```python
from build123d import *

# Parameters (mm, degrees)
SKIZZE1_W                       = 50
SKIZZE1_H                       = 2
SKIZZE1_W_2                     = 2
SKIZZE1_H_2                     = 48
AUFSATZ_LINEAR_AUSTRAGEN1_DEPTH = 30
AUFSATZ_LINEAR_AUSTRAGEN2_DEPTH = 30
SKIZZE3_R                       = 1.5
SCHNITT_LINEAR_AUSTRAGEN1_DEPTH = 30


with BuildPart() as part:
    # Skizze1 → Aufsatz-Linear austragen1 (new body)
    with BuildSketch(Plane.XY):
        with Locations((-2.795178436, 3.083333333)):
            Rectangle(SKIZZE1_W, SKIZZE1_H)
        with Locations((21.204821564, -21.916666667)):
            Rectangle(SKIZZE1_W_2, SKIZZE1_H_2)
    extrude(amount=AUFSATZ_LINEAR_AUSTRAGEN1_DEPTH)

    # Skizze2 → Aufsatz-Linear austragen2 (add)
    with BuildSketch(Plane.XY.offset(30)):
        Polygon((15.215533088, 2.083333333), (20.204821564, -2.916666667), (20.204821564, 2.083333333), align=None)
    extrude(amount=-AUFSATZ_LINEAR_AUSTRAGEN2_DEPTH)

    # Skizze3 → Schnitt-Linear austragen1 (cut)
    with BuildSketch(Plane(origin=(8.665746428, 8.647181758, 0), x_dir=(0, 0, 1), z_dir=(-0.7078646055315657, -0.7063481437900443, 0))):
        with Locations(Location((15, -12.806243307, 0), (0, 0, 270))):
            Circle(SKIZZE3_R)
    extrude(amount=-SCHNITT_LINEAR_AUSTRAGEN1_DEPTH, mode=Mode.SUBTRACT)


solid = part.part
```
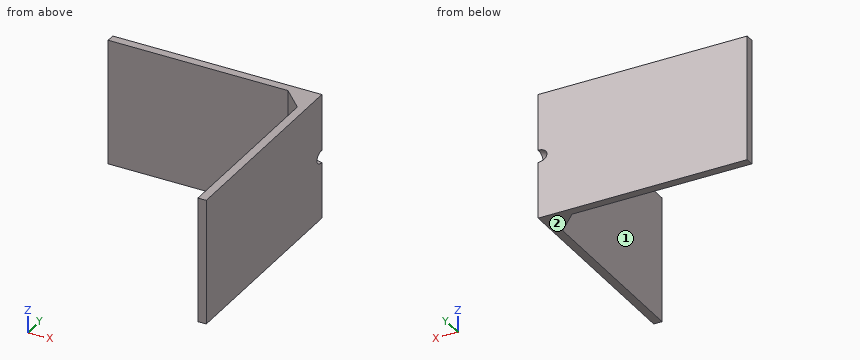
The model under review builds one solid part; all positions refer to its coordinate system, in mm. Face numbers are marked on the shaded views. A direction names the side the tool comes from. Round coordinates to 2 decimals unless told otherwise and drop trailing zeros. Write each loop counter-clockwise with the first axis right and the second up, starting at its lowest first coordinate (ties: lowest second). Pieces come first, ordered by that corner, then holes. Notation, with made-up numbers: (-15.75, 74.5) - (19.25, 74.5) arc R17 cw to (19.25, 87.5) - close; hole circle Ø9 at (52, 48.5). An arc over 180 degrees is marked (long way). One line per question, with ' | ' between items.
Item 1: For the marked faces 1 and 2, list the 3-axis set-ups (+Z, -Z, +X, -X, +Y, -Y) from which the entire face can be reached by the end or side of a thin tool; tool diameter is ignored.
Resolved:
face 1: +Z, -Z, -X, -Y | face 2: -Z, +X, -X, +Y, -Y
Item 2: Add section B-B, the plane y = -37. Give the boundary of the cut face in (x, z).
Resolved:
outline: (20.2, 0) - (22.2, 0) - (22.2, 30) - (20.2, 30) - close
Item 3: Add section C-C, the plane x = -1.5. Give the boundary of the cut face in (y, z).
Resolved:
outline: (2.08, 0) - (4.08, 0) - (4.08, 30) - (2.08, 30) - close
Item 4: To check wall thickness, follow probe 1 along Y at (x, z) = (15, 8); probe 2 along X at (y, z) = (-32, 26); probe 3 along X at (y, z) = (-0.5, 12). State the ranges of each line that lie inside material, in increasing order.
Resolved:
probe 1: y = 2.08 to 4.08 | probe 2: x = 20.2 to 22.2 | probe 3: x = 17.79 to 22.2
Item 5: Add section A-A, the plane z = 22.75. Give the boundary of the cut face in (x, y).
Resolved:
outline: (-27.8, 2.08) - (15.22, 2.08) - (20.2, -2.92) - (20.2, -45.92) - (22.2, -45.92) - (22.2, 4.08) - (-27.8, 4.08) - close
Item 6: For P1, Ø6, axis at x = -4, z = 19, coming from the -Y side; P2, Ø8, axis at y = -36.5, z = 17.5, coming from the -X side, all flat-tipped, find the tip position at first contact; note any pin that passes through.
Resolved:
P1: stops at y = 2.08 | P2: stops at x = 20.2
